For this review, take the finished solid that the model builds, in its own axes (mm). Face numbers are marked on the shaded views. A direction names the side the tool comes from. Coordinates: 2 decimals unless noted, no trailing zeros. Loops run counter-clockwise (first coordinate to the right, second up) from the corner with the lowest first, then second, coordinate; pieces in that order, holes last. Notation, with made-up numbers: (80.25, 25) - (98.25, 25) arc R27 ccw to (98.25, 53) - close; hole circle Ø4 at (62.5, 28). An arc over 180 degrees is marked (long way). Answer as a JSON object with one key per item and string values. Group by question number.
Item 1: Tool access review of the marked faces 1, 2 and 3: name each direction out of +Z, -Z, +X, -X, +Y, -Y from which nothing blocks a thin tool from reaching the whole face with its end or side.
Item 2: We need section A-A (z = 55). Give the boundary of the cut face in (x, y), then the cut area to 3 significant figures.
Item 3: Clearance check with flat-ended pins moving along their axes: pin 1 (5 mm diameter, centred on x = 5, z = 29, fed in from +Y); pin 2 (5 mm diameter, centred on x = -4, y = -14.5, fed in from +Z); pin 3 (8 mm diameter, centred on y = -23, z = 21, fed in from -X). State where each tip first meets the part, or that it passes through.
Item 4: We need section B-B (x = -3). Give the boundary of the cut face in (y, z), then the cut area to 3 significant figures.
Item 5: We need section D-D (x = -18). Give the boundary of the cut face in (y, z).
Item 6: To check wall thickness, follow line 1 (Y direction, x = -4.5, z = 25.5); line 2 (Z direction, x = -42, y = -26); line 3 (X direction, y = -26, z = 61.5). State the ranges of each line that lie inside material, in increasing order.
Item 7: We need section C-C (y = -30). Give the boundary of the cut face in (x, z).
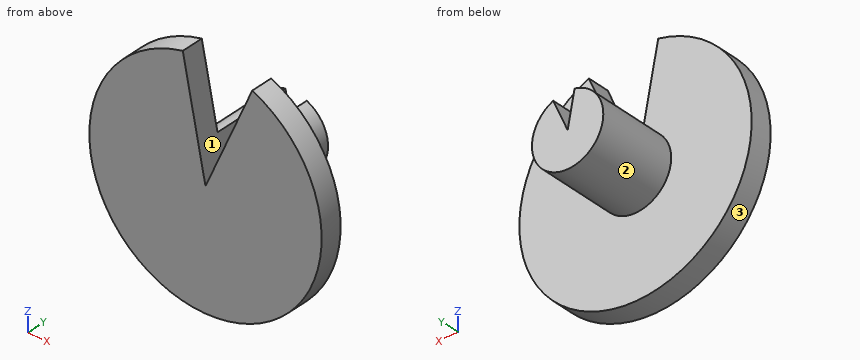
from build123d import *

# Parameters (mm, degrees)
F0_R     = 11
F1_DEPTH = 25
F2_R     = 35.80237
F3_DEPTH = 7
F5_DEPTH = 32.001


with BuildPart() as f1:
    # F0 (on Front) → F1 (new body)
    with BuildSketch(Plane.XZ):
        with Locations((-12.781085, 38.115203)):
            Circle(F0_R)
    extrude(amount=F1_DEPTH)

    # F2 (on face) → F3 (join)
    with BuildSketch(Plane.XZ.offset(25)):
        with Locations((-12.781085, 38.115203)):
            Circle(F2_R)
    extrude(amount=F3_DEPTH)

    # F4 (on face) → F5 (cut, through all)
    with BuildSketch(Plane.XZ.offset(32)):
        Polygon((-7.421601, 82.684956), (-19.784253, 73.225961), (-12.781085, 38.115203), (1.632773, 70.887911), align=None)
    extrude(amount=-F5_DEPTH, mode=Mode.SUBTRACT)


solid = f1.part
Check sheet entries:
{
 "1": {"face 1": "+Z, +Y, -Y", "face 2": "+Y", "face 3": "+Y, -Y"},
 "2": {"outline": "(-44.35, -32) - (-16.15, -32) - (-16.15, -25) - (-44.35, -25) - close; (-5.35, -32) - (18.79, -32) - (18.79, -25) - (-5.35, -25) - close", "area": "366 mm2"},
 "3": {"pin 1": "stops at y = -25", "pin 2": "stops at z = 47.15", "pin 3": "stops at x = -45.88"},
 "4": {"outline": "(-32, 3.67) - (-25, 3.67) - (-25, 33.08) - (0, 33.08) - (0, 43.15) - (-25, 43.15) - (-25, 60.35) - (-32, 60.35) - close", "area": "648 mm2"},
 "5": {"outline": "(-32, 2.7) - (-25, 2.7) - (-25, 28.43) - (0, 28.43) - (0, 47.8) - (-25, 47.8) - (-25, 64.28) - (-32, 64.28) - close"},
 "6": {"line 1": "y = -32 to -25", "line 2": "z = 17.43 to 58.8", "line 3": "x = -39.89 to -17.45, -2.5 to 14.33"},
 "7": {"outline": "(-19.78, 73.23) arc R35.8 ccw (long way) to (1.63, 70.89) - (-12.78, 38.12) - close"}
}
